Design review of the part shown in the three views and the two pictorial views. Dimensions are in mm from the part's minimum x, y and z. A direction names the side the tool comes from. Round coordinates to 2 decimals unless told otherwise and drop trailing zeros. Loops run counter-clockwise (first coordinate to the right, second up) from the corner with the lowest first, then second, coordinate; pieces in that order, holes last. Notation, with made-up numbers: (52.5, -31) - (94.5, -31) arc R12 ccw to (94.5, -27) - close; hole circle Ø1 at (-30, 55). An arc over 180 degrees is marked (long way). Return JSON: item names as keys, results as strings. Group by question number.
(1) Wall thickness on L1, parallel to Y at x = 29, z = 20.5; L2, parallel to X at y = 17.75, z = 11.75; L3, parallel to Z at x = 29.5, y = 23: over which ranges is each line inside the solid? List them lowest first. Write a range as [from, to].
(2) For the marked faces 1 and 2, list the 3-axis set-ups (+Z, -Z, +X, -X, +Y, -Y) from which the entire face can be reached by the end or side of a thin tool; tool diameter is ignored.
(3) The part is to be moulded in two halves that separate along X. For the marked faces 3, 4 and 5, say which applies: pulls with the +X half, pulls with the -X half, needs draft (parallel to the pull), parting line crosses it, or undercut.
(4) We need section C-C, the plane x = 18.5. Write out the cut boundary in (y, z).
(5) Clearance check with flat-ended pins moving along their axes: pin 1 (4 mm diameter, centred on x = 5, y = 24, fed in from +Z); pin 2 (1 mm diameter, centred on x = 11, y = 23, fed in from -Z). State where each tip first meets the part, or that it passes through.
(6) We need section A-A, the plane z = 11. Write out the cut boundary in (x, y), and give its area (3 significant figures).
(7) We need section D-D, the plane z = 19. Write out the cut boundary in (x, y), and give its area (3 significant figures).
(8) We need section B-B, the plane y = 12.5. Write out the cut boundary in (x, z).
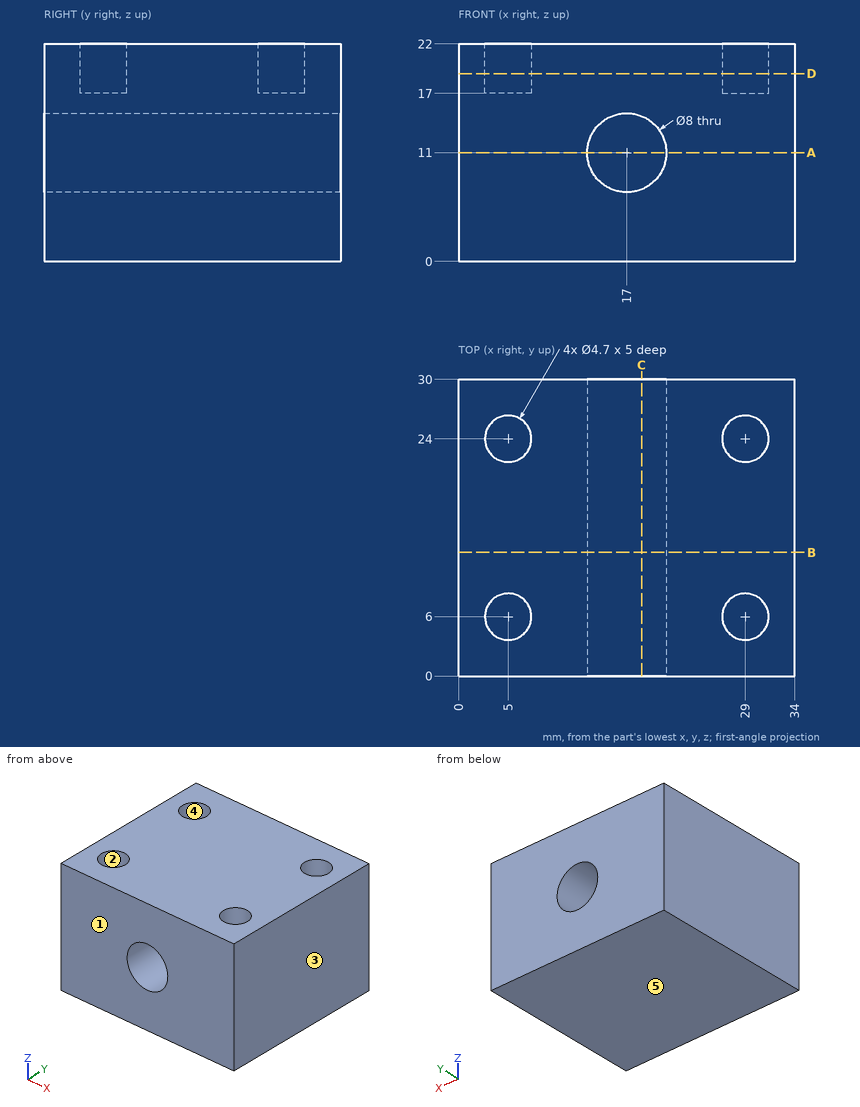
Solutions:
{
 "1": {"L1": "[0, 3.65], [8.35, 21.65], [26.35, 30]", "L2": "[0, 13.07], [20.93, 34]", "L3": "[0, 17]"},
 "2": {"face 1": "+Z, -Z, +X, -X, -Y", "face 2": "+Z"},
 "3": {"face 3": "pulls with the +X half", "face 4": "undercut", "face 5": "needs draft"},
 "4": {"outline": "(0, 0) - (30, 0) - (30, 7.29) - (0, 7.29) - close; (0, 14.71) - (30, 14.71) - (30, 22) - (0, 22) - close"},
 "5": {"pin 1": "z = 17", "pin 2": "z = 0"},
 "6": {"outline": "(0, 0) - (13, 0) - (13, 30) - (0, 30) - close; (21, 0) - (34, 0) - (34, 30) - (21, 30) - close", "area": "780 mm^2"},
 "7": {"outline": "(0, 0) - (34, 0) - (34, 30) - (0, 30) - close; hole circle Ø4.7 at (5, 6); hole circle Ø4.7 at (5, 24); hole circle Ø4.7 at (29, 6); hole circle Ø4.7 at (29, 24)", "area": "951 mm^2"},
 "8": {"outline": "(0, 0) - (34, 0) - (34, 22) - (0, 22) - close; hole circle Ø8 at (17, 11)"}
}
